For this review, take the finished solid that the model builds, in its own axes (mm). Coordinates: 2 decimals unless noted, no trailing zeros. Loops run counter-clockwise (first coordinate to the right, second up) from the corner with the lowest first, then second, coordinate; pieces in that order, holes last. Notation, with made-up numbers: (-22.75, -8.5) -> (26.25, -8.5) arc R11 ccw to (26.25, 7.5) -> close; hole circle Ø11 at (-8.75, 36). An arc over 180 degrees is marked (long way). One line per item, written item: value.
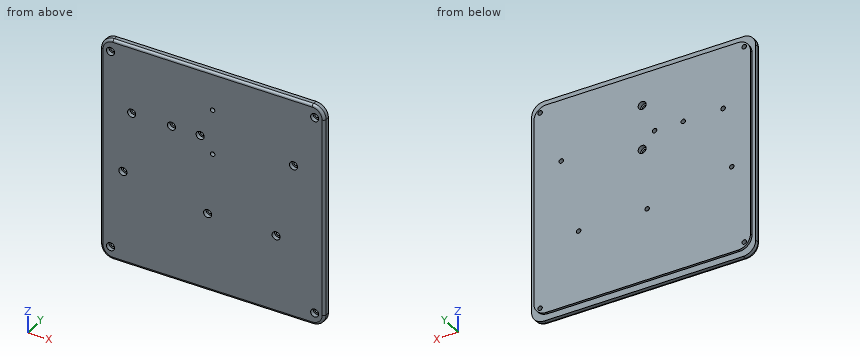
from build123d import *

# Parameters (mm, degrees)
SKIZZE1_W                                            = 180
SKIZZE1_H                                            = 180
AUFSATZ_LINEAR_AUSTRAGEN1_DEPTH                      = 5
AUFSATZ_LINEAR_AUSTRAGEN2_DEPTH                      = 2
STIRNSENKUNG_F_R_M3_ZYLINDERSCHRAUBE_MIT_D           = 3.6
STIRNSENKUNG_F_R_M3_ZYLINDERSCHRAUBE_MIT_DEPTH       = 9.1
STIRNSENKUNG_F_R_M3_ZYLINDERSCHRAUBE_MIT_CBORE_D     = 6.5
STIRNSENKUNG_F_R_M3_ZYLINDERSCHRAUBE_MIT_CBORE_DEPTH = 3.4
STIRNSENKUNG_F_R_M3_ZYLINDERSCHRAUBE_MIT_TIP         = 1.081549114
STIRNSENKUNG_F_R_M3_ZYLINDERSCHRAUBE_2_D             = 3.6
STIRNSENKUNG_F_R_M3_ZYLINDERSCHRAUBE_2_DEPTH         = 9.1
STIRNSENKUNG_F_R_M3_ZYLINDERSCHRAUBE_2_CBORE_D       = 6.5
STIRNSENKUNG_F_R_M3_ZYLINDERSCHRAUBE_2_CBORE_DEPTH   = 3.4
STIRNSENKUNG_F_R_M3_ZYLINDERSCHRAUBE_2_TIP           = 1.081549114
VERRUNDUNG1_R                                        = 10
VERRUNDUNG2_R                                        = 2
STIRNSENKUNG_F_R_M3_ZYLINDERSCHRAUBE_3_D             = 3.6
STIRNSENKUNG_F_R_M3_ZYLINDERSCHRAUBE_3_CBORE_D       = 6.5
STIRNSENKUNG_F_R_M3_ZYLINDERSCHRAUBE_3_CBORE_DEPTH   = 3.4


with BuildPart() as part:
    # Skizze1 → Aufsatz-Linear austragen1 (new body)
    with BuildSketch(Plane(origin=(0, 0, 0), x_dir=(1, 0, 0), z_dir=(0, 1, 0))):
        Rectangle(SKIZZE1_W, SKIZZE1_H)
    extrude(amount=AUFSATZ_LINEAR_AUSTRAGEN1_DEPTH)

    # Skizze2 → Aufsatz-Linear austragen2 (add)
    with BuildSketch(Plane(origin=(0, 5, 0), x_dir=(1, 0, 0), z_dir=(0, 1, 0))):
        with BuildLine():
            Line((77, 85), (-77, 85))
            ThreePointArc((-77, 85), (-84.071067812, 82.071067812), (-87, 75))
            Line((-87, 75), (-87, -75))
            ThreePointArc((-87, -75), (-84.071067812, -82.071067812), (-77, -85))
            Line((-77, -85), (77, -85))
            ThreePointArc((77, -85), (84.071067812, -82.071067812), (87, -75))
            Line((87, -75), (87, 75))
            ThreePointArc((87, 75), (84.071067812, 82.071067812), (77, 85))
        make_face()
    extrude(amount=AUFSATZ_LINEAR_AUSTRAGEN2_DEPTH)

    # Stirnsenkung f_r M3 Zylinderschraube mit
    with Locations(Plane(origin=(0, 7, 0), x_dir=(1, 0, 0), z_dir=(0, 1, 0))):
        with Locations((0, -23), (0, -59)):
            CounterBoreHole(STIRNSENKUNG_F_R_M3_ZYLINDERSCHRAUBE_MIT_D / 2, STIRNSENKUNG_F_R_M3_ZYLINDERSCHRAUBE_MIT_CBORE_D / 2, STIRNSENKUNG_F_R_M3_ZYLINDERSCHRAUBE_MIT_CBORE_DEPTH, depth=STIRNSENKUNG_F_R_M3_ZYLINDERSCHRAUBE_MIT_DEPTH)
            with Locations((0, 0, -(STIRNSENKUNG_F_R_M3_ZYLINDERSCHRAUBE_MIT_DEPTH + STIRNSENKUNG_F_R_M3_ZYLINDERSCHRAUBE_MIT_TIP / 2))):  # 118° drill point
                Cone(0, STIRNSENKUNG_F_R_M3_ZYLINDERSCHRAUBE_MIT_D / 2, STIRNSENKUNG_F_R_M3_ZYLINDERSCHRAUBE_MIT_TIP, mode=Mode.SUBTRACT)

    # Stirnsenkung f_r M3 Zylinderschraube 2
    with Locations(Plane(origin=(0, 0, 0), x_dir=(-1, 0, 0), z_dir=(0, -1, 0))):
        with Locations((-82, 80), (82, 80), (82, -80), (-82, -80)):
            CounterBoreHole(STIRNSENKUNG_F_R_M3_ZYLINDERSCHRAUBE_2_D / 2, STIRNSENKUNG_F_R_M3_ZYLINDERSCHRAUBE_2_CBORE_D / 2, STIRNSENKUNG_F_R_M3_ZYLINDERSCHRAUBE_2_CBORE_DEPTH, depth=STIRNSENKUNG_F_R_M3_ZYLINDERSCHRAUBE_2_DEPTH)
            with Locations((0, 0, -(STIRNSENKUNG_F_R_M3_ZYLINDERSCHRAUBE_2_DEPTH + STIRNSENKUNG_F_R_M3_ZYLINDERSCHRAUBE_2_TIP / 2))):  # 118° drill point
                Cone(0, STIRNSENKUNG_F_R_M3_ZYLINDERSCHRAUBE_2_D / 2, STIRNSENKUNG_F_R_M3_ZYLINDERSCHRAUBE_2_TIP, mode=Mode.SUBTRACT)

    # Verrundung1
    verrundung1_edges = [part.edges().sort_by_distance(p)[0] for p in [
        (90, 2.5, -90),
        (90, 2.5, 90),
        (-90, 2.5, 90),
        (-90, 2.5, -90),
    ]]
    fillet(verrundung1_edges, radius=VERRUNDUNG1_R)

    # Verrundung2
    verrundung2_edges = [part.edges().sort_by_distance(p)[0] for p in [
        (90, 0, 0),
        (0, 0, -90),
        (0, 0, 90),
        (-90, 0, 0),
        (87.071067812, 0, -87.071067812),
        (-87.071067812, 0, -87.071067812),
        (-87.071067812, 0, 87.071067812),
        (87.071067812, 0, 87.071067812),
    ]]
    fillet(verrundung2_edges, radius=VERRUNDUNG2_R)

    # Stirnsenkung f_r M3 Zylinderschraube 3 (through all)
    with Locations(Plane(origin=(0, 0, 0), x_dir=(-1, 0, 0), z_dir=(0, -1, 0))):
        with Locations((-51, 27), (4, 27), (-65, -35), (10, -35), (33, -35), (65, -35), (72, 15)):
            CounterBoreHole(STIRNSENKUNG_F_R_M3_ZYLINDERSCHRAUBE_3_D / 2, STIRNSENKUNG_F_R_M3_ZYLINDERSCHRAUBE_3_CBORE_D / 2, STIRNSENKUNG_F_R_M3_ZYLINDERSCHRAUBE_3_CBORE_DEPTH)


solid = part.part
1. Insertion check: pin 1 Ø2 at (x, z) = (-83.5, -78.5) entering from -Y; pin 2 Ø0.6 at (y, z) = (6.5, 26.5) entering from -X; pin 3 Ø6 at (x, z) = (0, 23) entering from +Y. Each pin has a flat end and moves straight along its axis. Give the tip position at first contact, or say it passes through.
Return value:
pin 1: stops at y = 3.4
pin 2: stops at x = -87
pin 3: stops at y = 3.6
2. To check wall thickness, follow probe 1 along X at (y, z) = (4.5, 80); probe 2 along Z at (x, y) = (65, 6.2); probe 3 along Z at (x, y) = (51, 2.35). State the ranges of each line that lie inside material, in increasing order. Write a range as from..to.
Return value:
probe 1: x = -90..-83.8, -80.2..80.2, 83.8..90
probe 2: z = -85..33.2, 36.8..85
probe 3: z = -90..-30.25, -23.75..90
3. Take a section at A-A, the plane x = -52.5. Give the boundary of the cut face in (y, z).
Return value:
outline: (0, -88) arc R2 ccw to (2, -90) -> (5, -90) -> (5, -85) -> (7, -85) -> (7, 85) -> (5, 85) -> (5, 90) -> (2, 90) arc R2 ccw to (0, 88) -> close
